Build history of the part. All positions in model axes, mm. Face numbers are marked on the shaded views. A direction names the side the tool comes from. Round coordinates to 2 decimals unless told otherwise and drop trailing zeros. Write each loop counter-clockwise with the first axis right and the second up, starting at its lowest first coordinate (ties: lowest second). Pieces come first, ordered by that corner, then holes. Notation, with made-up numbers: (36.25, 22.25) -> (45.25, 22.25) arc R13 cw to (45.25, 27.25) -> close; hole circle Ø1 at (-12, -21.5). An arc over 180 degrees is marked (long way). Return JSON: item names as keys, results as strings.
from build123d import *

# Parameters (mm, degrees)
SKETCH1_R                    = 10
BOSS_EXTRUDE1_DEPTH          = 75
SKETCH2_R                    = 15
BOSS_EXTRUDE2_DEPTH          = 10
SKETCH3_R                    = 2
CUT_EXTRUDE1_DEPTH           = 30
CUT_EXTRUDE1_TAPER           = 1
CUT_EXTRUDE1_OTHER_WAY_DEPTH = 30


with BuildPart() as part:
    # Sketch1 → Boss-Extrude1 (new body)
    with BuildSketch(Plane(origin=(0, 0, 0), x_dir=(1, 0, 0), z_dir=(0, 1, 0))):
        Circle(SKETCH1_R)
    extrude(amount=BOSS_EXTRUDE1_DEPTH)

    # Sketch2 → Boss-Extrude2 (add)
    with BuildSketch(Plane(origin=(0, 75, 0), x_dir=(1, 0, 0), z_dir=(0, 1, 0))):
        Circle(SKETCH2_R)
    extrude(amount=BOSS_EXTRUDE2_DEPTH)

    # Sketch3 → Cut-Extrude1 (cut)
    with BuildSketch(Plane.XY):
        with Locations((0, 10)):
            Circle(SKETCH3_R)
    extrude(amount=-CUT_EXTRUDE1_DEPTH, taper=CUT_EXTRUDE1_TAPER, mode=Mode.SUBTRACT)

    # Sketch3 → Cut-Extrude1 other way (cut)
    with BuildSketch(Plane.XY):
        with Locations((0, 10)):
            Circle(SKETCH3_R)
    extrude(amount=CUT_EXTRUDE1_OTHER_WAY_DEPTH, mode=Mode.SUBTRACT)


solid = part.part
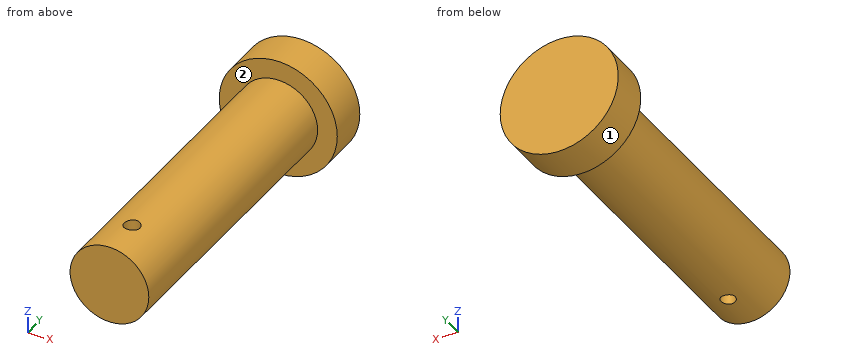
Q1. Pin check, flat tips, straight feed: pin 1 Ø3 at (x, y) = (-4, 51) entering from +Z; pin 2 Ø5 at (x, y) = (0, 10) entering from +Z; pin 3 Ø3 at (y, z) = (67.5, 8) entering from +X; pin 4 Ø5 at (y, z) = (73.5, 1) entering from +X. Stop position of each tip, or through.
Verdict:
{"pin 1": "stops at z = 9.68", "pin 2": "stops at z = 10", "pin 3": "stops at x = 7.6", "pin 4": "stops at x = 15"}
Q2. Saw through at A-A on x = 8.5. List the corners of the cut face in (y, z), then the cut area to 3 significant figures.
Verdict:
{"outline": "(0, -5.27) -> (75, -5.27) -> (75, -12.36) -> (85, -12.36) -> (85, 12.36) -> (75, 12.36) -> (75, 5.27) -> (0, 5.27) -> close", "area": "1,040 mm²"}
Q3. Saw through at B-B on y = 47. List the corners of the cut face in (x, z).
Verdict:
{"outline": "circle Ø20 at (0, 0)"}
Q4. Wall check: L1, parallel to Y at x = 0, z = 7.5; L2, parallel to X at y = 9, z = -1; L3, parallel to Y at x = 11, z = -0.5. Give the ranges that are in metal, low to high.
Verdict:
{"L1": "y = 0 to 8, 12 to 85", "L2": "x = -9.95 to -1.71, 1.71 to 9.95", "L3": "y = 75 to 85"}
Q5. Saw through at D-D on x = 3. List the corners of the cut face in (y, z).
Verdict:
{"outline": "(0, -9.54) -> (75, -9.54) -> (75, -14.7) -> (85, -14.7) -> (85, 14.7) -> (75, 14.7) -> (75, 9.54) -> (0, 9.54) -> close"}
Q6. Saw through at C-C on z = -11.25. List the corners of the cut face in (x, y), then the cut area to 3 significant figures.
Verdict:
{"outline": "(-9.92, 75) -> (9.92, 75) -> (9.92, 85) -> (-9.92, 85) -> close", "area": "198 mm²"}
Q7. 3-axis set-ups, long thin cutter, end or side, ignore diameter. For the marked faces 1 and 2: which of +Z, -Z, +X, -X, +Y, -Y reach the whole face in a straight line?
Verdict:
{"face 1": "+Y, -Y", "face 2": "-Y"}
